Input: part model. Units: mm. Frame: model coordinates. Give positions to 0.01 mm unless a question says otherwise; leave off trailing zeros. Loops run counter-clockwise (first coordinate to the right, second up) from the corner with the lowest first, then second, coordinate; pieces in that order, holes last. Notation, with made-up numbers: (-38, -13) -> (-4, -13) arc R30 cw to (-4, 24) -> close; hole circle Ø6 at (-25.5, 12.5). An arc over 180 degrees is marked (long way). Answer as a JSON object with one key per item and string values.
```python
from build123d import *

# Parameters (mm, degrees)
SKETCH_1_R      = 28
SKETCH_1_R_2    = 25
EXTRUDE_1_DEPTH = 2
SKETCH_2_W      = 1.809411118
SKETCH_2_H      = 1.819947288
SKETCH_2_W_2    = 1.819947288
SKETCH_2_H_2    = 1.809411118
EXTRUDE_2_DEPTH = 1


with BuildPart() as part:
    # 草图1 → 凸台-拉伸1 (new body)
    with BuildSketch(Plane(origin=(0, 0, 0), x_dir=(1, 0, 0), z_dir=(0, 1, 0))):
        with Locations(Location((0, 0, 0), (0, 0, 270))):
            Circle(SKETCH_1_R)
        with Locations(Location((0, 0, 0), (0, 0, 270))):
            Circle(SKETCH_1_R_2, mode=Mode.SUBTRACT)
    extrude(amount=EXTRUDE_1_DEPTH)

    # 草图2 → 凸台-拉伸2 (add)
    with BuildSketch(Plane(origin=(0, 2, 0), x_dir=(1, 0, 0), z_dir=(0, 1, 0))):
        Polygon((7.587666599, 26.280125266), (9.308518833, 25.720986481), (8.746124192, 23.990113753), (7.025271959, 24.549252538), align=None)
        with Locations((0, 26.428628666)):
            Rectangle(SKETCH_2_W, SKETCH_2_H)
        Polygon((15.337305084, 22.649166456), (16.801149428, 21.585621286), (15.731411252, 20.113253001), (14.267566908, 21.176798171), align=None)
        Polygon((21.585621286, 16.801149428), (22.649166456, 15.337305084), (21.176798171, 14.267566908), (20.113253001, 15.731411252), align=None)
        Polygon((25.720986481, 9.308518833), (26.280125266, 7.587666599), (24.549252538, 7.025271959), (23.990113753, 8.746124192), align=None)
        with Locations((26.428628666, 0)):
            Rectangle(SKETCH_2_W_2, SKETCH_2_H_2)
        Polygon((26.280125266, -7.587666599), (25.720986481, -9.308518833), (23.990113753, -8.746124192), (24.549252538, -7.025271959), align=None)
        Polygon((22.649166456, -15.337305084), (21.585621286, -16.801149428), (20.113253001, -15.731411252), (21.176798171, -14.267566908), align=None)
        Polygon((16.801149428, -21.585621286), (15.337305084, -22.649166456), (14.267566908, -21.176798171), (15.731411252, -20.113253001), align=None)
        Polygon((9.308518833, -25.720986481), (7.587666599, -26.280125266), (7.025271959, -24.549252538), (8.746124192, -23.990113753), align=None)
        with Locations((0, -26.428628666)):
            Rectangle(SKETCH_2_W, SKETCH_2_H)
        Polygon((-7.587666599, -26.280125266), (-9.308518833, -25.720986481), (-8.746124192, -23.990113753), (-7.025271959, -24.549252538), align=None)
        Polygon((-15.337305084, -22.649166456), (-16.801149428, -21.585621286), (-15.731411252, -20.113253001), (-14.267566908, -21.176798171), align=None)
        Polygon((-21.585621286, -16.801149428), (-22.649166456, -15.337305084), (-21.176798171, -14.267566908), (-20.113253001, -15.731411252), align=None)
        Polygon((-25.720986481, -9.308518833), (-26.280125266, -7.587666599), (-24.549252538, -7.025271959), (-23.990113753, -8.746124192), align=None)
        with Locations((-26.428628666, 0)):
            Rectangle(SKETCH_2_W_2, SKETCH_2_H_2)
        Polygon((-26.280125266, 7.587666599), (-25.720986481, 9.308518833), (-23.990113753, 8.746124192), (-24.549252538, 7.025271959), align=None)
        Polygon((-22.649166456, 15.337305084), (-21.585621286, 16.801149428), (-20.113253001, 15.731411252), (-21.176798171, 14.267566908), align=None)
        Polygon((-16.801149428, 21.585621286), (-15.337305084, 22.649166456), (-14.267566908, 21.176798171), (-15.731411252, 20.113253001), align=None)
        Polygon((-9.308518833, 25.720986481), (-7.587666599, 26.280125266), (-7.025271959, 24.549252538), (-8.746124192, 23.990113753), align=None)
    extrude(amount=EXTRUDE_2_DEPTH)


solid = part.part
```
Q1. Section B-B, the plane z = 11.5. Return the cut outline in (x, y).
Evaluation:
{"outline": "(-25.53, 0) -> (-22.2, 0) -> (-22.2, 2) -> (-25.53, 2) -> close; (22.2, 0) -> (25.53, 0) -> (25.53, 2) -> (22.2, 2) -> close"}
Q2. Section D-D, the plane z = 0. Return the cut outline in (x, y).
Evaluation:
{"outline": "(-28, 0) -> (-25, 0) -> (-25, 2) -> (-25.52, 2) -> (-25.52, 3) -> (-27.34, 3) -> (-27.34, 2) -> (-28, 2) -> close; (25, 0) -> (28, 0) -> (28, 2) -> (27.34, 2) -> (27.34, 3) -> (25.52, 3) -> (25.52, 2) -> (25, 2) -> close"}
Q3. Section A-A, the plane x = 0. Return the cut outline in (y, z), then the cut area to 3 significant figures.
Evaluation:
{"outline": "(0, -28) -> (2, -28) -> (2, -27.34) -> (3, -27.34) -> (3, -25.52) -> (2, -25.52) -> (2, -25) -> (0, -25) -> close; (0, 25) -> (2, 25) -> (2, 25.52) -> (3, 25.52) -> (3, 27.34) -> (2, 27.34) -> (2, 28) -> (0, 28) -> close", "area": "15.6 mm2"}
Q4. Section C-C, the plane y = 0.45. Return the cut outline in (x, z), then the cut area to 3 significant figures.
Evaluation:
{"outline": "circle Ø56 at (0, 0); hole circle Ø50 at (0, 0)", "area": "500 mm2"}
Q5. Pin query (flat end, axial travel): pin 1 (0.8 mm diameter, centred on x = -0.5, y = 2.5, fed in from -Z); pin 2 (0.5 mm diameter, centred on x = 0.5, y = 2.5, fed in from +Z); pin 3 (1 mm diameter, centred on y = 2, z = -10.5, fed in from +X); pin 4 (8 mm diameter, centred on x = 17, z = -9.5, fed in from -Y). Return the tip coordinate at first contact, or that it passes through.
Evaluation:
{"pin 1": "stops at z = -27.34", "pin 2": "stops at z = 27.34", "pin 3": "stops at x = 26.15", "pin 4": "passes through"}
Q6. Draft query along Z for faces 1 (the flat face through (11, 2, -23)), 2 (the flat face through (-16, 3, 21)), 3 (the cylindrical face through (-27.334, 0.986, -6.07)). Return one class per face: +Z half, -Z half, draft (parallel to the pull), parting line (faces both ways), or undercut.
Evaluation:
{"face 1": "undercut", "face 2": "draft", "face 3": "parting line"}
Q7. Ray query, line 1 along X through (y, z) = (0.9, 0); line 2 along Y through (x, z) = (-18, -19.5); line 3 along X through (y, z) = (2.35, 8.5). Return the intervals inside material, ascending.
Evaluation:
{"line 1": "x = -28 to -25, 25 to 28", "line 2": "y = 0 to 2", "line 3": "x = -25.98 to -24.07, 24.07 to 25.98"}
